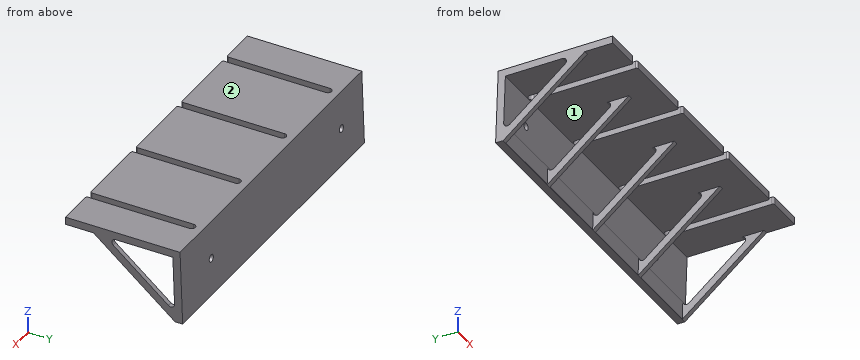
```python
from build123d import *

# Parameters (mm, degrees)
F1_DEPTH = 4
F4_DEPTH = 176
F6_W     = 40.25
F6_H     = 35.9756330808
F6_W_2   = 41.5
F7_REACH = 113.8761797882
F8_R     = 2
F9_DEPTH = 25


# Not quite as in the source:
# - a feature names something its author has since deleted; it is built from what else it names


with BuildPart() as f1:
    # F0 (on Top) → F1 (new body)
    with BuildSketch(Plane.XY):
        with BuildLine():
            Line((176, 0), (0, 0))
            Line((0, 0), (0, -61.56))
            Line((0, -61.56), (19, -61.56))
            ThreePointArc((19, -61.56), (19.7071067812, -61.2671067812), (20, -60.56))
            Line((20, -60.56), (20, -6))
            ThreePointArc((20, -6), (22, -4), (24, -6))
            Line((24, -6), (24, -60.56))
            ThreePointArc((24, -60.56), (24.2928932188, -61.2671067812), (25, -61.56))
            Line((25, -61.56), (63, -61.56))
            ThreePointArc((63, -61.56), (63.7071067812, -61.2671067812), (64, -60.56))
            Line((64, -60.56), (64, -6))
            ThreePointArc((64, -6), (66, -4), (68, -6))
            Line((68, -6), (68, -60.56))
            ThreePointArc((68, -60.56), (68.2928932188, -61.2671067812), (69, -61.56))
            Line((69, -61.56), (107, -61.56))
            ThreePointArc((107, -61.56), (107.7071067812, -61.2671067812), (108, -60.56))
            Line((108, -60.56), (108, -6))
            ThreePointArc((108, -6), (110, -4), (112, -6))
            Line((112, -6), (112, -60.56))
            ThreePointArc((112, -60.56), (112.2928932188, -61.2671067812), (113, -61.56))
            Line((113, -61.56), (151, -61.56))
            ThreePointArc((151, -61.56), (151.7071067812, -61.2671067812), (152, -60.56))
            Line((152, -60.56), (152, -6))
            ThreePointArc((152, -6), (154, -4), (156, -6))
            Line((156, -6), (156, -60.56))
            ThreePointArc((156, -60.56), (156.2928932188, -61.2671067812), (157, -61.56))
            Line((157, -61.56), (176, -61.56))
            Line((176, -61.56), (176, 0))
        make_face()
    extrude(amount=F1_DEPTH)

    # F3 (on face) → F4 (join, through all)
    with BuildSketch(Plane(origin=(0, 0, 0), x_dir=(0, -1, 0), z_dir=(-1, 0, 0))):
        with BuildLine():
            Line((2.9423112754, -26.3580624732), (3.8627550992, 0))
            Line((3.8627550992, 0), (0, 0))
            Line((0, 0), (0, 4))
            Line((0, 4), (-1.3959798681, -35.9756330808))
            Line((-1.3959798681, -35.9756330808), (2.60158344, -36.1152310676))
            Line((2.60158344, -36.1152310676), (46.56, 0))
            Line((46.56, 0), (34.6739806412, 0))
            ThreePointArc((34.6739806412, 0), (36.5568879354, -1.3257151036), (35.9435965909, -3.5453398785))
            Line((35.9435965909, -3.5453398785), (6.2107088791, -27.9732013451))
            ThreePointArc((6.2107088791, -27.9732013451), (4.0550404197, -28.220878742), (2.9423112754, -26.3580624732))
        make_face()
    extrude(amount=-F4_DEPTH)

    f7_end = Plane(origin=(88, -3.299573374, -16.1274145272), x_dir=(0, -0.0348994967, 0.999390827), z_dir=(0, 0.999390827, 0.0348994967))
    # F6 (on face) → F7 (cut, up to a plane its end follows)
    with BuildSketch(Plane.XZ.offset(61.56)):
        with Locations((153.375, -17.9878165404)):
            Rectangle(F6_W, F6_H)
        with Locations((110, -17.9878165404)):
            Rectangle(F6_W_2, F6_H)
        with Locations((66, -17.9878165404)):
            Rectangle(F6_W_2, F6_H)
        Polygon((19, 0), (2.5, 0), (2.5, -35.9756330808), (42.75, -35.9756330808), (42.75, 0), align=None)
    f7_long = extrude(amount=-F7_REACH, mode=Mode.PRIVATE)
    add(split(f7_long, bisect_by=f7_end, keep=Keep.BOTTOM, mode=Mode.PRIVATE), mode=Mode.SUBTRACT)

    # F8 (on face) → F9 (cut)
    with BuildSketch(Plane(origin=(0, 0.1395129475, 0.0048718995), x_dir=(-1, 0, 0), z_dir=(0, 0.999390827, 0.0348994967))):
        with Locations((-147.0000000001, -16.0024366919)):
            Circle(F8_R)
        with Locations((-21, -16.0024366919)):
            Circle(F8_R)
    extrude(amount=-F9_DEPTH, mode=Mode.SUBTRACT)


solid = f1.part
```
Geometry check sheet. Reference: the model listing, model coordinates, mm. Face numbers are marked on the shaded views. Round coordinates to 2 decimals unless told otherwise and drop trailing zeros. Order: outer loops, then holes, each group sorted by start corner. A loop starts at its lowest first (then second) coordinate and runs counter-clockwise, first axis right, second up. Notation, with made-up numbers: M 14.5,80.5 L 30.5,80.5 A20 cw 30.5,94.5 Z; hole C -39,24 d4. An arc over 180 degrees is marked long. Answer as CSV lines item,"result".
1) Sectioned sample at B-B on z = -10.5. Record the cut outline in (x, y).
Entries:
outline,"M 0,-33.78 L 2.5,-33.78 L 2.5,-27.48 L 0,-27.48 Z; M 0,-3.5 L 176,-3.5 L 176,0.51 L 0,0.51 Z; M 42.75,-33.78 L 45.25,-33.78 L 45.25,-27.48 L 42.75,-27.48 Z; M 86.75,-33.78 L 89.25,-33.78 L 89.25,-27.48 L 86.75,-27.48 Z; M 130.75,-33.78 L 133.25,-33.78 L 133.25,-27.48 L 130.75,-27.48 Z; M 173.5,-33.78 L 176,-33.78 L 176,-27.48 L 173.5,-27.48 Z"
2) Thickness scan on probe 1 along X at (y, z) = (-22, -19); probe 2 along Z at (x, y) = (127.5, -33); probe 3 along Z at (x, y) = (110, -2). Record the ranges inside material, lowest first. Write a range as [from, to].
Entries:
probe 1,"[0, 2.5], [42.75, 45.25], [86.75, 89.25], [130.75, 133.25], [173.5, 176]"
probe 2,"[0, 4]"
probe 3,"[-36.09, 4]"
3) Mould release check, pull along X, two halves, no side actions. Record for the marked faces 1 and 2: +X half, -X half, draft (parallel to the pull), parting line (faces both ways), or undercut.
Entries:
face 1,"undercut"
face 2,"draft"
4) Sectioned sample at C-C on x = 51.5. Record the cut outline in (y, z).
Entries:
outline,"M -61.56,0 L -3.86,0 L -2.61,-35.98 L -2.77,-35.98 L -2.6,-36.12 L 1.4,-35.98 L 0,4 L -61.56,4 Z"
5) Sectioned sample at D-D on x = 110. Record the cut outline in (y, z), and give its area (3 significant figures).
Entries:
outline,"M -4,0 L -3.86,0 L -2.61,-35.98 L -2.77,-35.98 L -2.6,-36.12 L 1.4,-35.98 L 0,4 L -4,4 Z"
area,"161 mm2"
6) Gauge pin test, flat ends, axial feed: pin 1 Ø1 at (x, z) = (126.5, -27.5) entering from +Y; pin 2 Ø8 at (x, z) = (138, -13) entering from -Y; pin 3 Ø1.2 at (y, z) = (-36.5, 2) entering from -X; pin 4 Ø1 at (x, z) = (99.5, -6) entering from -Y. Record the tip position at first contact, or that the pin passes through.
Entries:
pin 1,"y = 1.12"
pin 2,"y = -3.55"
pin 3,"x = 0"
pin 4,"y = -3.67"
7) Sectioned sample at A-A on y = -52. Record the cut outline in (x, z), and give its area (3 significant figures).
Entries:
outline,"M 0,0 L 20,0 L 20,4 L 0,4 Z; M 24,0 L 64,0 L 64,4 L 24,4 Z; M 68,0 L 108,0 L 108,4 L 68,4 Z; M 112,0 L 152,0 L 152,4 L 112,4 Z; M 156,0 L 176,0 L 176,4 L 156,4 Z"
area,"640 mm2"
